The listing builds one solid part. Answer for the finished solid, in the listing's coordinates (mm). Give positions to 0.01 mm unless a question says otherwise; leave off trailing zeros. Write each loop counter-clockwise with the first axis right and the second up, starting at its lowest first coordinate (ties: lowest second). Pieces come first, ordered by that corner, then holes. Notation, with made-up numbers: (65, -25) -> (123, -25) arc R23 ccw to (123, -7) -> close; hole circle Ø8 at (15.25, 31.5). An arc over 180 degrees is marked (long way). Put each result on its own line as item: value. Start each with the question number.
1) A cutting plane is placed at C-C (y = 2.5). Write down the section's boundary in (x, z).
2) A cutting plane is placed at B-B (x = 42.5). Write down the section's boundary in (y, z) (3 decimals), then the cut area to 3 significant figures.
3) A cutting plane is placed at A-A (z = -25). Write down the section's boundary in (x, y) (3 decimals).
4) A flat-ended cylindrical pin translates along its axis: pin 1 Ø5 at (x, z) = (5, -5) entering from -Y. Find the tip coordinate at first contact, or state that the pin passes through.
5) Find the intervals of material crossed by line 1 along X through (y, z) = (2.3, -105); line 2 along Z through (x, y) = (57, 2.3); line 3 along X through (y, z) = (2.1, -55), in increasing order. Write a range as from..to.
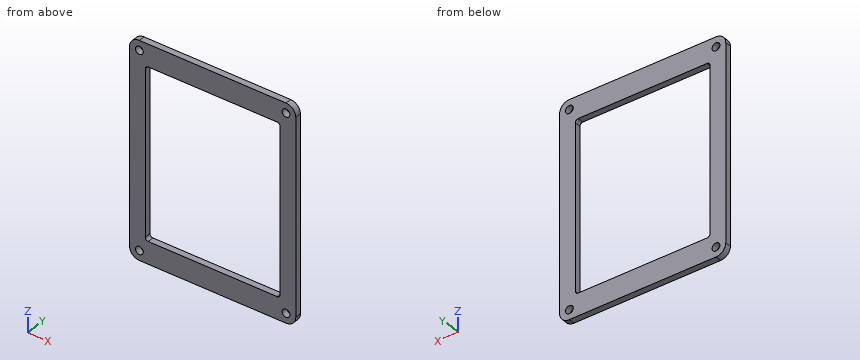
from build123d import *

# Parameters (mm, degrees)
SKETCH1_W           = 85
SKETCH1_H           = 110
BOSS_EXTRUDE1_DEPTH = 3.175
FILLET1_R           = 5
SKETCH3_W           = 68.982
SKETCH3_H           = 87.204
CUT_EXTRUDE3_DEPTH  = 140.050640506
FILLET2_R           = 1.5
SKETCH5_R           = 2
CUT_EXTRUDE4_DEPTH  = 140.050640506


with BuildPart() as part:
    # Sketch1 → Boss-Extrude1 (new body)
    with BuildSketch(Plane(origin=(0, 0, 0), x_dir=(1, 0, 0), z_dir=(0, 1, 0))):
        with Locations((42.5, 55)):
            Rectangle(SKETCH1_W, SKETCH1_H)
    extrude(amount=BOSS_EXTRUDE1_DEPTH)

    # Fillet1
    fillet1_edges = [part.edges().sort_by_distance(p)[0] for p in [
        (0, 1.5875, -110),
        (85, 1.5875, -110),
        (85, 1.5875, 0),
        (0, 1.5875, 0),
    ]]
    fillet(fillet1_edges, radius=FILLET1_R)

    # Sketch3 → Cut-Extrude3 (cut, through all)
    with BuildSketch(Plane(origin=(0, 3.175, 0), x_dir=(1, 0, 0), z_dir=(0, 1, 0))):
        with Locations((42.5, 55)):
            Rectangle(SKETCH3_W, SKETCH3_H)
    extrude(amount=-CUT_EXTRUDE3_DEPTH, mode=Mode.SUBTRACT)

    # Fillet2
    fillet2_edges = [part.edges().sort_by_distance(p)[0] for p in [
        (76.991, 1.5875, -98.602),
        (76.991, 1.5875, -11.398),
        (8.009, 1.5875, -11.398),
        (8.009, 1.5875, -98.602),
    ]]
    fillet(fillet2_edges, radius=FILLET2_R)

    # Sketch5 → Cut-Extrude4 (cut, through all)
    with BuildSketch(Plane(origin=(0, 3.175, 0), x_dir=(1, 0, 0), z_dir=(0, 1, 0))):
        with Locations(Location((5, 5, 0), (0, 0, 270))):
            Circle(SKETCH5_R)
        with Locations(Location((80, 5, 0), (0, 0, 270))):
            Circle(SKETCH5_R)
        with Locations(Location((80, 105, 0), (0, 0, 270))):
            Circle(SKETCH5_R)
        with Locations(Location((5, 105, 0), (0, 0, 270))):
            Circle(SKETCH5_R)
    extrude(amount=-CUT_EXTRUDE4_DEPTH, mode=Mode.SUBTRACT)


solid = part.part
Reply:
1. outline: (0, -105) arc R5 ccw to (5, -110) -> (80, -110) arc R5 ccw to (85, -105) -> (85, -5) arc R5 ccw to (80, 0) -> (5, 0) arc R5 ccw to (0, -5) -> close; hole circle Ø4 at (5, -105); hole circle Ø4 at (5, -5); hole (8.01, -97.1) arc R1.5 ccw to (9.51, -98.6) -> (75.49, -98.6) arc R1.5 ccw to (76.99, -97.1) -> (76.99, -12.9) arc R1.5 ccw to (75.49, -11.4) -> (9.51, -11.4) arc R1.5 ccw to (8.01, -12.9) -> close; hole circle Ø4 at (80, -105); hole circle Ø4 at (80, -5)
2. outline: (0, -110) -> (3.175, -110) -> (3.175, -98.602) -> (0, -98.602) -> close; (0, -11.398) -> (3.175, -11.398) -> (3.175, 0) -> (0, 0) -> close
2. area: 72.4 mm2
3. outline: (0, 0) -> (8.009, 0) -> (8.009, 3.175) -> (0, 3.175) -> close; (76.991, 0) -> (85, 0) -> (85, 3.175) -> (76.991, 3.175) -> close
4. pin 1: stops at y = 0
5. line 1: x = 0..3, 7..78, 82..85
5. line 2: z = -110..-98.6, -11.4..0
5. line 3: x = 0..8.01, 76.99..85
